from build123d import *

# Parameters (mm, degrees)
F0_R     = 6.35
F0_R_2   = 3.175
F1_DEPTH = 6.35
F2_R     = 0.762
F4_D     = 3.175


with BuildPart() as f1:
    # F0 (on Top) → F1 (new body)
    with BuildSketch(Plane.XY):
        with BuildLine():
            ThreePointArc((-15.4277360093, -33.1291600779), (-17.6097258518, -31.6297541594), (-19.7516389471, -30.0736352458))
            Line((-19.7516389471, -30.0736352458), (-20.0273010704, -31.3041983899))
            ThreePointArc((-20.0273010704, -31.3041983899), (-15.605527233, -43.9673113737), (-2.2926258159, -45.6022946054))
            Line((-2.2926258159, -45.6022946054), (3.3420161223, -42.9899532533))
            ThreePointArc((3.3420161223, -42.9899532533), (-0.5573553186, -41.3437618471), (-4.3842812821, -39.5355357964))
            ThreePointArc((-4.3842812821, -39.5355357964), (-9.1948370721, -40.2356556442), (-13.0909002079, -37.32837051))
            ThreePointArc((-13.0909002079, -37.32837051), (-14.2898816566, -35.2457737279), (-15.4277360093, -33.1291600779))
        make_face()
        with BuildLine():
            ThreePointArc((5.8890733938, 11.2520582367), (-4.6857632411, 11.8039664032), (-12.0029711474, 4.1495401716))
            ThreePointArc((-12.0029711474, 4.1495401716), (-9.4049707621, -13.9914505961), (-2.1779859288, -30.8323485013))
            ThreePointArc((-2.1779859288, -30.8323485013), (-1.4791469298, -35.6407535094), (-4.3842812821, -39.5355357964))
            ThreePointArc((-4.3842812821, -39.5355357964), (-0.5573553186, -41.3437618471), (3.3420161223, -42.9899532533))
            Line((3.3420161223, -42.9899532533), (31.8875731001, -29.7556182717))
            Line((31.8875731001, -29.7556182717), (36.2849774034, -27.7168869328))
            ThreePointArc((36.2849774034, -27.7168869328), (43.6394950275, -16.5000431331), (36.8322335447, -4.9428935964))
            Line((36.8322335447, -4.9428935964), (5.8890733938, 11.2520582367))
        make_face()
        Circle(F0_R, mode=Mode.SUBTRACT)
        with BuildLine():
            ThreePointArc((37.2931601509, -16.1949518331), (35.5866457226, -20.5262959369), (31.384328105, -22.5296081644))
            ThreePointArc((31.384328105, -22.5296081644), (26.2996745793, -11.8636077292), (37.2931601509, -16.1949518331))
        make_face(mode=Mode.SUBTRACT)
        with BuildLine():
            ThreePointArc((-18.7919287035, -25.7894628669), (-17.199620286, -29.5004662895), (-15.4277360093, -33.1291600779))
            ThreePointArc((-15.4277360093, -33.1291600779), (-10.0074027219, -36.507133329), (-4.3842812821, -39.5355357964))
            ThreePointArc((-4.3842812821, -39.5355357964), (-1.4791469298, -35.6407535094), (-2.1779859288, -30.8323485013))
            ThreePointArc((-2.1779859288, -30.8323485013), (-9.4049707621, -13.9914505961), (-12.0029711474, 4.1495401716))
            ThreePointArc((-12.0029711474, 4.1495401716), (-12.2172281013, 3.4683335365), (-12.3928580021, 2.7761611158))
            Line((-12.3928580021, 2.7761611158), (-18.7919287035, -25.7894628669))
        make_face()
        with Locations((-7.6344430684, -34.0803595057)):
            Circle(F0_R_2, mode=Mode.SUBTRACT)
        with BuildLine():
            Line((-18.7919287035, -25.7894628669), (-19.7516389471, -30.0736352458))
            ThreePointArc((-19.7516389471, -30.0736352458), (-17.6097258518, -31.6297541594), (-15.4277360093, -33.1291600779))
            ThreePointArc((-15.4277360093, -33.1291600779), (-17.199620286, -29.5004662895), (-18.7919287035, -25.7894628669))
        make_face()
        with BuildLine():
            ThreePointArc((-4.3842812821, -39.5355357964), (-10.0074027219, -36.507133329), (-15.4277360093, -33.1291600779))
            ThreePointArc((-15.4277360093, -33.1291600779), (-14.2898816566, -35.2457737279), (-13.0909002079, -37.32837051))
            ThreePointArc((-13.0909002079, -37.32837051), (-9.1948370721, -40.2356556442), (-4.3842812821, -39.5355357964))
        make_face()
        with Locations((-7.6344430684, -34.0803595057)):
            Circle(F0_R_2)
    extrude(amount=F1_DEPTH)

    # F2
    f2_edges = [f1.edges().sort_by_distance(p)[0] for p in [
        (-15.605527, -43.967311, 6.35),
        (16.996176, -36.659591, 6.35),
        (16.996176, -36.659591, 0),
        (-15.605527, -43.967311, 0),
    ]]
    fillet(f2_edges, radius=F2_R)

    # F4 (through all)
    with Locations(Plane.XY.offset(6.35)):
        with Locations((-7.6344430684, -34.0803595057)):
            Hole(F4_D / 2)


solid = f1.part
Read the model definition and answer for the solid it produces. Units are mm, in the model's axes. Give positions to 0.01 mm unless a question says otherwise; leave off trailing zeros. Answer in a Markdown table with one row per item. Add a question column.
Item 1: Find the intervals of material crossed by L1, parallel to Y at x = 26.5, z = 3.25; L2, parallel to Y at x = 0, z = 4; L3, parallel to X at y = -3, z = 0.75, in increasing order.
Item 2: Flat-ended cylindrical pins translate along their axes: P1, Ø1.5, axis at y = 3.5, z = 5.5, coming from the +X side; P2, Ø1.5, axis at y = 2.5, z = 5, coming from the -X side; P3, Ø3, axis at y = -11, z = 2.5, coming from the +X side. Find the tip coordinate at first contact, or state that the pin passes through.
Item 3: Section A-A, the plane z = 2 is taken. Count the separate pieces of the cut face and the enclosed holes in it, and give its area (3 significant figures).
Item 4: Determine the mould class of faces 1 (the face through (-6.46, -33.01, 3.13)), 2 (the face through (-1.38, -6.2, 3.13)), 3 (the face through (43.633, -16.698, 3.141)), 4 (the face through (21.04, 3.08, 6.12)) for opening direction Y: pulls with the +Y half, pulls with the -Y half, needs draft (parallel to the pull), parting line crosses it, or undercut.
Recorded:
| question | item | result |
|---|---|---|
| 1 | L1 | y = -32.25 to -20.73, -11.66 to 0.46 |
| 1 | L2 | y = -44.54 to -6.35, 6.35 to 12.7 |
| 1 | L3 | x = -13.69 to -5.6, 5.6 to 33.12 |
| 2 | P1 | stops at x = 22.13 |
| 2 | P2 | stops at x = -12.62 |
| 2 | P3 | stops at x = 43.09 |
| 3 | separate pieces | 1 |
| 3 | enclosed holes | 3 |
| 3 | area | 2,260 mm2 |
| 4 | face 1 | undercut |
| 4 | face 2 | undercut |
| 4 | face 3 | parting line crosses it |
| 4 | face 4 | pulls with the +Y half |
